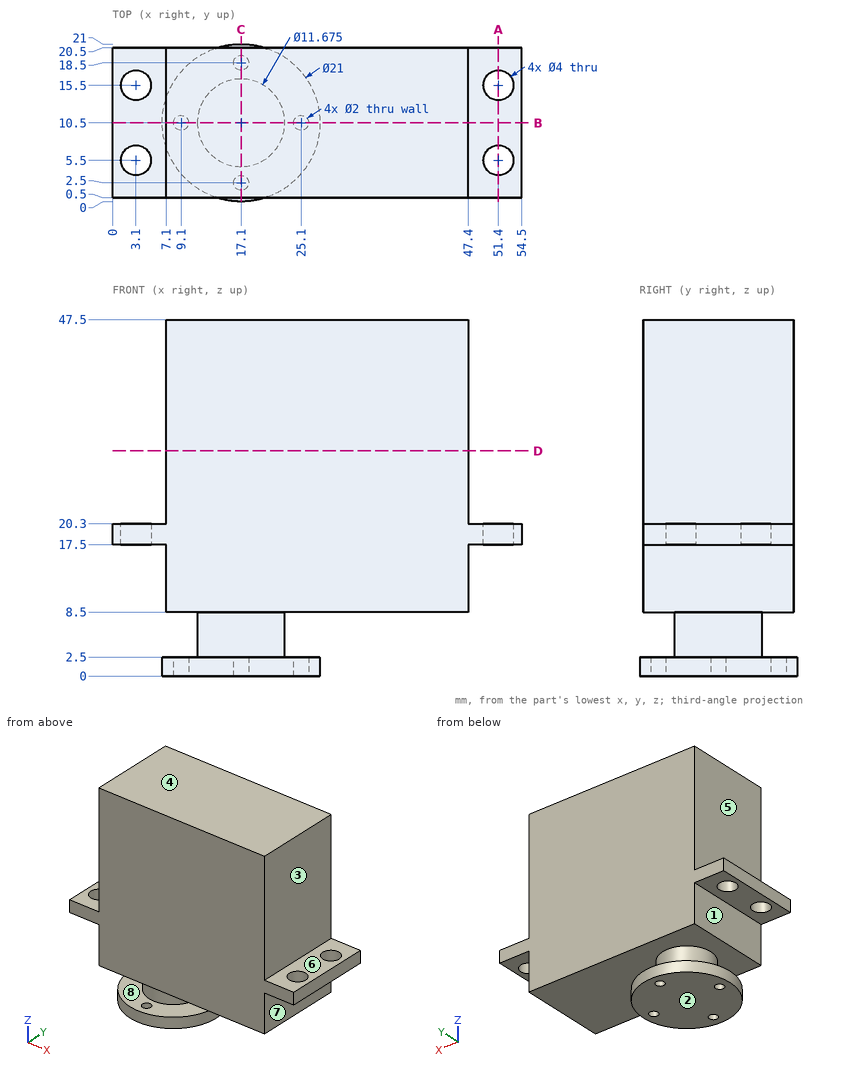
The drawing under review shows one solid part. Ordinate dimensions are in mm from its lowest x, y, z. A direction names the side the tool comes from. Coordinates: 2 decimals unless noted, no trailing zeros. Write each loop counter-clockwise with the first axis right and the second up, starting at its lowest first coordinate (ties: lowest second). Pieces come first, ordered by that corner, then holes. Notation, with made-up numbers: M 73.5,-32 L 127.5,-32 A15 cw 127.5,-27 Z; hole C 6.25,14 d4. An arc over 180 degrees is marked long. Answer as a JSON object with one key per item and string values.
Item 1: Draft analysis for pull direction Z (two halves, no side actions). For the marked faces 1, 2, 3 and 4, state which applies: pulls with the +Z half, pulls with the -Z half, needs draft (parallel to the pull), parting line crosses it, or undercut.
Outcome:
{"face 1": "undercut", "face 2": "pulls with the -Z half", "face 3": "needs draft", "face 4": "pulls with the +Z half"}
Item 2: Machinability: for the marked faces 5, 6, 7 and 8, which of the approach directions +Z, -Z, +X, -X, +Y, -Y give a long, thin tool a straight path to every point of the face, cutting with its end or side? Answer none if there is none.
Outcome:
{"face 5": "+Z, -X, +Y, -Y", "face 6": "+Z, +X, +Y, -Y", "face 7": "-Z, +X, +Y, -Y", "face 8": "none"}
Item 3: Add section A-A, the plane x = 51.4. Give the boundary of the cut face in (y, z), and give its area (3 significant figures).
Outcome:
{"outline": "M 0.5,17.5 L 3.5,17.5 L 3.5,20.3 L 0.5,20.3 Z; M 7.5,17.5 L 13.5,17.5 L 13.5,20.3 L 7.5,20.3 Z; M 17.5,17.5 L 20.5,17.5 L 20.5,20.3 L 17.5,20.3 Z", "area": "33.6 mm²"}
Item 4: Add section D-D, the plane z = 30. Give the boundary of the cut face in (x, y).
Outcome:
{"outline": "M 7.1,0.5 L 47.4,0.5 L 47.4,20.5 L 7.1,20.5 Z"}
Item 5: Wall thickness on probe 1 along Y at (x, z) = (17, 1) (1 decimal); probe 2 along Z at (x, y) = (10.5, 16); probe 3 along Z at (x, y) = (2, 10.5): over which ranges is each line inside the solid? List them lowest first.
Outcome:
{"probe 1": "0 to 1.5, 3.5 to 17.5, 19.5 to 21", "probe 2": "0 to 2.5, 8.5 to 47.5", "probe 3": "17.5 to 20.3"}
Item 6: Insertion check: pin 1 Ø3.5 at (x, y) = (3.1, 5.5) entering from -Z; pin 2 Ø12 at (x, z) = (14, 31) entering from -Y; pin 3 Ø4.5 at (y, z) = (5.5, 11) entering from +X; pin 4 Ø5.5 at (x, y) = (2, 11.5) entering from +Z. Each pin has a flat end and moves straight along its axis. Give the tip position at first contact, or say it passes through.
Outcome:
{"pin 1": "through", "pin 2": "y = 0.5", "pin 3": "x = 47.4", "pin 4": "z = 20.3"}
Item 7: Add section C-C, the plane x = 17.1. Give the boundary of the cut face in (y, z).
Outcome:
{"outline": "M 0,0 L 1.5,0 L 1.5,2.5 L 0,2.5 Z; M 0.5,8.5 L 4.66,8.5 L 4.66,2.5 L 3.5,2.5 L 3.5,0 L 17.5,0 L 17.5,2.5 L 16.34,2.5 L 16.34,8.5 L 20.5,8.5 L 20.5,47.5 L 0.5,47.5 Z; M 19.5,0 L 21,0 L 21,2.5 L 19.5,2.5 Z"}
Item 8: Add section B-B, the plane y = 10.5. Give the boundary of the cut face in (x, z).
Outcome:
{"outline": "M 0,17.5 L 7.1,17.5 L 7.1,8.5 L 11.26,8.5 L 11.26,2.5 L 10.1,2.5 L 10.1,0 L 24.1,0 L 24.1,2.5 L 22.94,2.5 L 22.94,8.5 L 47.4,8.5 L 47.4,17.5 L 54.5,17.5 L 54.5,20.3 L 47.4,20.3 L 47.4,47.5 L 7.1,47.5 L 7.1,20.3 L 0,20.3 Z; M 6.6,0 L 8.1,0 L 8.1,2.5 L 6.6,2.5 Z; M 26.1,0 L 27.6,0 L 27.6,2.5 L 26.1,2.5 Z"}
